Autodesk Inventor part; units mm, degrees
ref_plane "YZ Plane" through (0, 0, 0) normal (1, 0, 0) x (0, 1, 0)
ref_plane "XZ Plane" through (0, 0, 0) normal (0, 1, 0) x (-1, 0, 0)
ref_plane "XY Plane" through (0, 0, 0) normal (0, 0, 1) x (1, 0, 0)
sketch "Sketch1" plane through (0, 0, 0) normal (0, 1, 0) x (-1, 0, 0)
  line L0 (1.2588, 13) -> (7.9588, 13)
  line L1 (7.9588, 13) -> (7.9588, 0)
  line L2 (7.9588, 0) -> (1.2588, 0)
  line L3 (1.2588, 0) -> (1.2588, 13)
  line L4 (7.9588, 1.0722) -> (10.1386, 14.0497)
  line L5 (10.1386, 14.0497) -> (9.9588, 14.0799)
  line L6 (9.9588, 14.0799) -> (7.9588, 2.173)
  point P0 (0, 0)
  dimension "d0" = 13
  dimension "d1" = 6.7
  dimension "d2" = 2
extrude "Extrusion1" add sketch "Sketch1" along normal blind 6 contours L0 L1 L2 L3
extrude "Extrusion2" add sketch "Sketch1" along normal blind 6 contours L6 L5 L4 L1
properties part number "koncnostikalo"
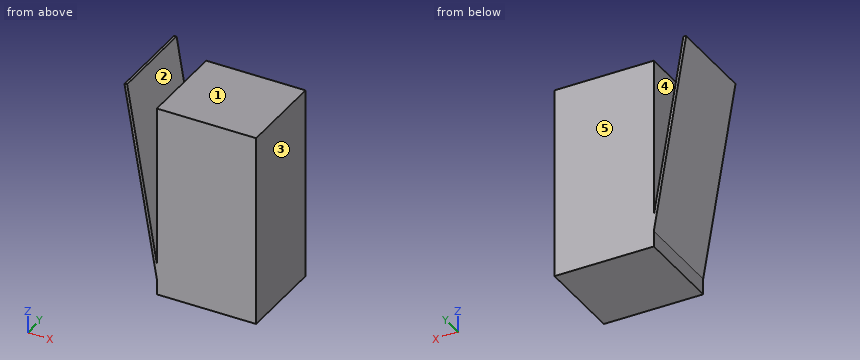
Here's how the part is built. I have some questions about the finished solid (model axes, mm). Face numbers are marked on the shaded views. A direction names the side the tool comes from. Give positions to 0.01 mm unless a question says otherwise; leave off trailing zeros. Order: outer loops, then holes, each group sorted by start corner. A loop starts at its lowest first (then second) coordinate and runs counter-clockwise, first axis right, second up. Notation, with made-up numbers: (80, -32.75) - (122, -32.75) arc R18 ccw to (122, -13.75) - close; hole circle Ø9 at (75.25, 42.25). An arc over 180 degrees is marked (long way). Answer as a JSON object with one key per item and string values. Group by question number.
Item 1: Which directions (+Z, -Z, +X, -X, +Y, -Y) give clear straight access to the entire face, cutting with the end or side of a thin tool? Please do the marked faces 4 and 5.
Item 2: If we mould it in two halves opening along X, with no side actions, what happens to the marked faces 1, 2 and 3? For each: pulls with the +X half, pulls with the -X half, needs draft (parallel to the pull), parting line crosses it, or undercut.
Item 3: If we section it at C-C on x = -5.75: Please give me the cut outline in (y, z).
Item 4: Please list where these lines run through material, in increasing order: probe 1 along Z at (x, y) = (-2.25, 5.15); probe 2 along X at (y, z) = (3.75, 9); probe 3 along X at (y, z) = (2.55, 4.75).
Item 5: If we section it at A-A on y = 4.25: Please give me the cut outline in (x, z).
Item 6: If we section it at D-D on x = -9.25: Please give me the cut outline in (y, z).
Item 7: For P1, Ø0.5, axis at y = 2, z = 0.5, coming from the -X side; P2, Ø1, axis at y = 1.5, z = 11.5, coming from the -X side, each with a flat end and sliding along its axis, tell me the tip position at first contact or that it passes through.
Item 8: If we section it at B-B on z = 4.25: Please give me the cut outline in (x, y), and give its area (3 significant figures).
Result set:
{
 "1": {"face 4": "+Z, +Y, -Y", "face 5": "+Z, -Z, +X, -X, +Y"},
 "2": {"face 1": "needs draft", "face 2": "undercut", "face 3": "pulls with the +X half"},
 "3": {"outline": "(0, 0) - (6, 0) - (6, 13) - (0, 13) - close"},
 "4": {"probe 1": "0 to 13", "probe 2": "-9.29 to -9.11, -7.96 to -1.26", "probe 3": "-8.58 to -8.39, -7.96 to -1.26"},
 "5": {"outline": "(-10.14, 14.05) - (-7.96, 1.07) - (-7.96, 0) - (-1.26, 0) - (-1.26, 13) - (-7.96, 13) - (-7.96, 2.17) - (-9.96, 14.08) - close"},
 "6": {"outline": "(0, 8.76) - (6, 8.76) - (6, 9.86) - (0, 9.86) - close"},
 "7": {"P1": "x = -7.96", "P2": "x = -9.79"},
 "8": {"outline": "(-8.49, 0) - (-8.31, 0) - (-8.31, 6) - (-8.49, 6) - close; (-7.96, 0) - (-1.26, 0) - (-1.26, 6) - (-7.96, 6) - close", "area": "41.3 mm²"}
}
